```python
from build123d import *

# Parameters (mm, degrees)
SKETCH_3_R      = 1.5
EXTRUDE_1_DEPTH = 1
SKETCH_1_R      = 1.5
EXTRUDE_2_DEPTH = 1
SKETCH_4_W      = 65
SKETCH_4_H      = 12
EXTRUDE_3_DEPTH = 1


with BuildPart() as part:
    # Sketch 3 → Extrude 1 (new body)
    with BuildSketch(Plane.XY.offset(10)):
        with BuildLine():
            Line((-26.8, 8.010393038), (-36.190694621, 8.96898207))
            ThreePointArc((-36.190694621, 8.96898207), (-42.7999991, 2.996713251), (-36.184155472, -2.968310943))
            Line((-36.184155472, -2.968310943), (-26.8, -2))
            Line((-26.8, -2), (43.2, -2))
            Line((43.2, -2), (43.2, 8.010393038))
            Line((43.2, 8.010393038), (-26.8, 8.010393038))
        make_face()
        with Locations((33.2, 3)):
            Circle(SKETCH_3_R, mode=Mode.SUBTRACT)
        with Locations((-11.8, 3)):
            Circle(SKETCH_3_R, mode=Mode.SUBTRACT)
        with Locations((-21.8, 3)):
            Circle(SKETCH_3_R, mode=Mode.SUBTRACT)
        with Locations((-36.8, 3)):
            Circle(SKETCH_3_R, mode=Mode.SUBTRACT)
    extrude(amount=EXTRUDE_1_DEPTH)



with BuildPart() as body_2:
    # Sketch 1 → Extrude 2 (new body)
    with BuildSketch(Plane.XY):
        with BuildLine():
            Line((43.2, 8.010393038), (-26.8, 8.010393038))
            Line((-26.8, 8.010393038), (-36.190694621, 8.96898207))
            ThreePointArc((-36.190694621, 8.96898207), (-42.7999991, 2.996713251), (-36.184155472, -2.968310943))
            Line((-36.184155472, -2.968310943), (-26.8, -2))
            Line((-26.8, -2), (43.2, -2))
            Line((43.2, -2), (43.2, 8.010393038))
        make_face()
        with Locations((-36.8, 3)):
            Circle(SKETCH_1_R, mode=Mode.SUBTRACT)
        with Locations((-21.8, 3)):
            Circle(SKETCH_1_R, mode=Mode.SUBTRACT)
        with Locations((-11.8, 3)):
            Circle(SKETCH_1_R, mode=Mode.SUBTRACT)
        with Locations((33.2, 3)):
            Circle(SKETCH_1_R, mode=Mode.SUBTRACT)
    extrude(amount=-EXTRUDE_2_DEPTH)


with BuildPart() as part_1:
    add(part.part)

    add(body_2.part)  # Extrude 3 merges body 2
    # Sketch 4 → Extrude 3 (add)
    with BuildSketch(Plane.XZ.offset(2)):
        with Locations((10.7, 5)):
            Rectangle(SKETCH_4_W, SKETCH_4_H)
    extrude(amount=EXTRUDE_3_DEPTH)


solid = part_1.part
```
CAD build for the part. Positions are in the model's coordinates, mm. Coordinates: 2 decimals unless noted, no trailing zeros. Order: outer loops, then holes, each group sorted by start corner. A loop starts at its lowest first (then second) coordinate and runs counter-clockwise, first axis right, second up. Notation, with made-up numbers: (5, 32) - (21, 32) arc R27 ccw to (21, 53) - close; hole circle Ø10 at (49, -6.75). An arc over 180 degrees is marked (long way). Use a Markdown table: item, result. Add a question column.
(1) Pull direction X, two halves, no side cores. Call faces 1 (the face through (-23.3, 3.07, -0.49)), 2 (the face through (-23.3, 3.07, 10.49)), 3 (the face through (43.2, -2.4, 5)), 4 (the face through (10, -2, 5)): +X half, -X half, draft (parallel to the pull), parting line (faces both ways), or undercut.
(2) Flat gauge pins, fed straight in: pin 1 (5 mm diameter, centred on x = 8, z = 6, fed in from +Y); pin 2 (3 mm diameter, centred on y = 6.5, z = 9, fed in from -X); pin 3 (0.8 mm diameter, centred on y = -2.5, z = 6.5, fed in from -X). Where does each tip first touch, or does it go through?
(3) Saw through at D-D (x = 11.5). Give the cut face in (y, z), then the cut area to 3 significant figures.
(4) Saw through at A-A (x = 33.2). Give the cut face in (y, z).
(5) Drill centre lines: line 1 along Z through (x, y) = (-17.5, 0); line 2 along Y through (x, z) = (-36.8, -0.5); line 3 along Y through (x, z) = (31.5, 4). Where is each one in solid material? Low to high. Write a range as [from, to].
(6) Saw through at B-B (y = 6.25). Give the cut face in (x, z).
(7) Saw through at C-C (x = -33). Give the cut face in (y, z), then the cut area to 3 significant figures.
Solved:
| question | item | result |
|---|---|---|
| 1 | face 1 | undercut |
| 1 | face 2 | undercut |
| 1 | face 3 | +X half |
| 1 | face 4 | draft |
| 2 | pin 1 | stops at y = -2 |
| 2 | pin 2 | stops at x = -42.31 |
| 2 | pin 3 | stops at x = -21.8 |
| 3 | outline | (-3, -1) - (8.01, -1) - (8.01, 0) - (-2, 0) - (-2, 10) - (8.01, 10) - (8.01, 11) - (-3, 11) - close |
| 3 | area | 32.0 mm² |
| 4 | outline | (-3, -1) - (1.5, -1) - (1.5, 0) - (-2, 0) - (-2, 10) - (1.5, 10) - (1.5, 11) - (-3, 11) - close; (4.5, -1) - (8.01, -1) - (8.01, 0) - (4.5, 0) - close; (4.5, 10) - (8.01, 10) - (8.01, 11) - (4.5, 11) - close |
| 5 | line 1 | z = [-1, 0], [10, 11] |
| 5 | line 2 | y = [-3, 1.5], [4.5, 9] |
| 5 | line 3 | y = [-3, -2] |
| 6 | outline | (-41.84, -1) - (43.2, -1) - (43.2, 0) - (-41.84, 0) - close; (-41.84, 10) - (43.2, 10) - (43.2, 11) - (-41.84, 11) - close |
| 7 | outline | (-2.64, -1) - (8.64, -1) - (8.64, 0) - (-2.64, 0) - close; (-2.64, 10) - (8.64, 10) - (8.64, 11) - (-2.64, 11) - close |
| 7 | area | 22.6 mm² |
